Could you check a few things on this model? Use its own coordinates, in mm. A direction names the side the tool comes from. Give positions to 0.01 mm unless a question says otherwise; leave off trailing zeros. Loops run counter-clockwise (first coordinate to the right, second up) from the corner with the lowest first, then second, coordinate; pieces in that order, holes last. Notation, with made-up numbers: (-22.75, 25.5) - (-5.75, 25.5) arc R17 cw to (-5.75, 29.5) - close; hole circle Ø6 at (-5.75, 37.25). An arc over 180 degrees is marked (long way). One line per item, written item: value. Start each with the question number.
Q1. I want a section at B-B (y = 4). Please give me the cut outline in (x, z), then the cut area to 3 significant figures.
Q2. For faces 1 (the face through (6, 4, -1)), 2 (the face through (1.7, 4, 6)), 3 (the face through (-1.916, 5.455, 7.148)), 4 (the face through (-6, 4, 1.7)), 5 (the face through (1, 4, 6)), which set-ups out of +Z, -Z, +X, -X, +Y, -Y let a thin tool reach every point of the face, with its end or its side?
Q3. If I drill on line 1 (Z direction, x = 1.25, y = 3.7); line 2 (Y direction, x = -5.5, z = -3.75); line 3 (Z direction, x = 0.75, y = 1.4), over which ranges is the centre line in solid material (lowest first)? Write a range as from..to.
Q4. I want a section at A-A (z = 0). Please give me the cut outline in (x, y), then the cut area to 3 significant figures.
Q5. I want a section at C-C (x = 0). Please give me the cut outline in (y, z).
Q6. I want a section at D-D (y = 0.8). Please give me the cut outline in (x, z), then the cut area to 3 significant figures.
Q7. I'm going to push flat-ended pins straight in: P1, Ø1.4, axis at y = 3.5, z = 6.5, coming from the -X side; P2, Ø0.5, axis at x = -6, y = 4, coming from the -Z side; P3, Ø1.1, axis at y = 3.5, z = -6.5, coming from the -X side; P4, Ø3, axis at x = 0, z = 0, coming from the -Y side. Where does each tip first touch, or does it pass through?
Q8. If we mould it in two halves opening along X, with no side actions, what happens to faces 6 (the face through (-1, 4, -6)), 7 (the face through (1.216, 2.859, -1.115)), 8 (the face through (-1.7, 4, -6)), 9 (the face through (-6, 4, 1))? For each: released by +X, released by -X, zero draft, split by the parting line, or undercut.
```python
from build123d import *

# Parameters (mm, degrees)
TROU_TARAUD_M41_D            = 3.3
TROU_TARAUD_M41_DEPTH        = 11.5
TROU_TARAUD_M41_TIP          = 0.991420021
ESQUISSE4_W                  = 5.010008652
ESQUISSE4_H                  = 3.395361839
ESQUISSE4_W_2                = 3.395361839
ESQUISSE4_H_2                = 5.010008652
ENL_V_MAT_EXTRU_1_DEPTH      = 10
BOSS_EXTRU_1_DEPTH           = 0.7
R_P_TITION_CIRCULAIRE1_COUNT = 4


with BuildPart() as part:
    # Esquisse1 → Révolution1 (revolve)
    with BuildSketch(Plane.XY, mode=Mode.PRIVATE) as r_volution1_sk:
        Polygon((0, 0), (2.5, 0), (2.5, 5.1), (7.4, 5.1), (7.4, 5.8), (0, 5.8), align=None)
    revolve(r_volution1_sk.sketch.rotate(Axis((0, 0, 0), (0, 1, 0)), 90), axis=Axis((0, 0, 0), (0, 1, 0)))

    # Trou taraudé M41
    with Locations(Plane(origin=(0, 5.8, 0), x_dir=(1, 0, 0), z_dir=(0, 1, 0))):
        with Locations((0, 0)):
            Hole(TROU_TARAUD_M41_D / 2, depth=TROU_TARAUD_M41_DEPTH)
            with Locations((0, 0, -(TROU_TARAUD_M41_DEPTH + TROU_TARAUD_M41_TIP / 2))):  # 118° drill point
                Cone(0, TROU_TARAUD_M41_D / 2, TROU_TARAUD_M41_TIP, mode=Mode.SUBTRACT)

    # Esquisse4 → Enlèv. mat.-Extru.1 (cut)
    with BuildSketch(Plane(origin=(0, 5.8, 0), x_dir=(1, 0, 0), z_dir=(0, 1, 0))):
        with Locations((4.205004326, -6.69768092)):
            Rectangle(ESQUISSE4_W, ESQUISSE4_H)
        with Locations((6.69768092, 4.205004326)):
            Rectangle(ESQUISSE4_W_2, ESQUISSE4_H_2)
        with Locations((-6.69768092, -4.205004326)):
            Rectangle(ESQUISSE4_W_2, ESQUISSE4_H_2)
        with Locations((-4.205004326, 6.69768092)):
            Rectangle(ESQUISSE4_W, ESQUISSE4_H)
    extrude(amount=-ENL_V_MAT_EXTRU_1_DEPTH, mode=Mode.SUBTRACT)

    # Esquisse5 → Boss.-Extru.1 (add)
    with BuildSketch(Plane(origin=(0, 0, -1.7), x_dir=(-1, 0, 0), z_dir=(0, 0, -1))):
        with BuildLine():
            Line((-5.369357503, 1), (-5.369357503, 5.8))
            Line((-5.369357503, 5.8), (-7.202083032, 5.8))
            ThreePointArc((-7.202083032, 5.8), (-6.728319202, 3.23100784), (-5.369357503, 1))
        make_face()
    boss_extru_1 = extrude(amount=-BOSS_EXTRU_1_DEPTH)

    # Répétition circulaire1: Boss.-Extru.1 ×4 about axis
    r_p_tition_circulaire1_axis = Axis((0, 0, 0), (0, 1, 0))
    for i in range(1, R_P_TITION_CIRCULAIRE1_COUNT):
        add(boss_extru_1.rotate(r_p_tition_circulaire1_axis, i * 360 / R_P_TITION_CIRCULAIRE1_COUNT))


solid = part.part
```
Worked answers:
1. outline: (-6.97, 1) - (-5.37, 1) - (-5.37, 1.7) - (-6.97, 1.7) - close; circle Ø5 at (0, 0); (-1.7, -6.97) - (-1, -6.97) - (-1, -5.37) - (-1.7, -5.37) - close; (1, 5.37) - (1.7, 5.37) - (1.7, 6.97) - (1, 6.97) - close; (5.37, -1.7) - (6.97, -1.7) - (6.97, -1) - (5.37, -1) - close; hole circle Ø3.3 at (0, 0)
1. area: 15.6 mm²
2. face 1: +Z, +X, -Y
2. face 2: +Z, +X, +Y, -Y
2. face 3: +Z, +Y, -Y
2. face 4: +Z, -X, +Y, -Y
2. face 5: +Z, -X, -Y
3. line 1: z = -2.17..-1.08, 1.08..2.17, 5.37..6.89
3. line 2: y = 5.1..5.8
3. line 3: z = -2.38..-1.47, 1.47..2.38
4. outline: (-7.4, 5.1) - (-2.5, 5.1) - (-2.5, 0) - (-1.65, 0) - (-1.65, 5.8) - (-7.4, 5.8) - close; (1.65, 0) - (2.5, 0) - (2.5, 5.1) - (7.4, 5.1) - (7.4, 5.8) - (1.65, 5.8) - close
4. area: 16.7 mm²
5. outline: (0, -2.5) - (5.1, -2.5) - (5.1, -7.4) - (5.8, -7.4) - (5.8, -1.65) - (0, -1.65) - close; (0, 1.65) - (5.8, 1.65) - (5.8, 7.4) - (5.1, 7.4) - (5.1, 2.5) - (0, 2.5) - close
6. outline: circle Ø5 at (0, 0); hole circle Ø3.3 at (0, 0)
6. area: 11.1 mm²
7. P1: stops at x = 1
7. P2: stops at z = 1
7. P3: stops at x = -1.7
7. P4: passes through
8. face 6: released by +X
8. face 7: undercut
8. face 8: released by -X
8. face 9: zero draft
